The figure shows three views and two pictorial views of one solid part (mm, origin at its lowest corner). Answer the questions. Give positions to 0.01 mm unless a question says otherwise; leave off trailing zeros. Loops run counter-clockwise (first coordinate to the right, second up) from the corner with the lowest first, then second, coordinate; pieces in that order, holes last. Notation, with made-up numbers: (69, 48.5) - (93, 48.5) arc R15 ccw to (93, 57.5) - close; hole circle Ø6 at (-24.75, -21). An arc over 180 degrees is marked (long way). Use a Markdown table: item, result. Add a question column.
Item 1: Consider probe 1 along Y at (x, z) = (10, 2.05); probe 2 along X at (y, z) = (6, 1.15); probe 3 along X at (y, z) = (5.5, 0.45). Determine where each line is inside the solid, lowest interval first. Write a range as [from, to].
Item 2: A cutting plane is placed at B-B (y = 1.5). Determine the outline of the cut face in (x, z), plus the area to 3 significant figures.
Item 3: This flat-tipped pin is pushed along its axis until it touches: P1, Ø1, axis at y = 8, z = 4, coming from the -X side. Where does it stop, or does it pass through?
Item 4: A cutting plane is placed at C-C (x = 10). Determine the outline of the cut face in (y, z), plus the area to 3 significant figures.
Item 5: A cutting plane is placed at A-A (z = 2.5). Determine the outline of the cut face in (x, y), plus the area to 3 significant figures.
Item 6: A cutting plane is placed at D-D (y = 4.85). Determine the outline of the cut face in (x, z), plus the area to 3 significant figures.
Item 7: For a pull along Y with two mould halves and no side action, classify the marked faces 1, 2, 3 and 4 as +Y half, -Y half, draft (parallel to the pull), parting line (faces both ways), or undercut.
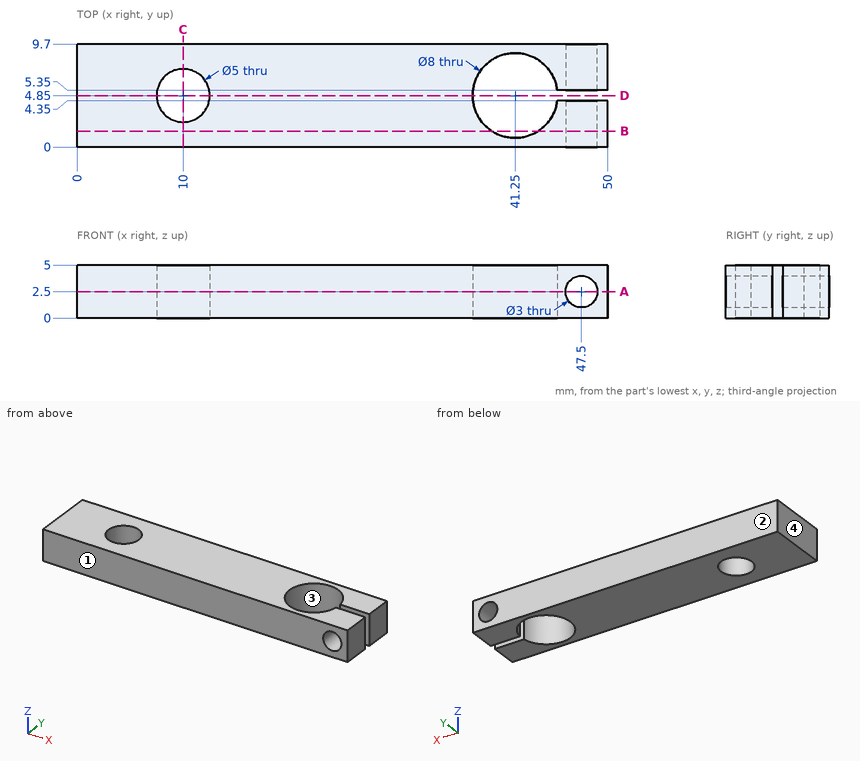
Geometry says:
| question | item | result |
|---|---|---|
| 1 | probe 1 | [0, 2.35], [7.35, 9.7] |
| 1 | probe 2 | [0, 7.78], [12.22, 37.42], [45.08, 46.85], [48.15, 50] |
| 1 | probe 3 | [0, 7.59], [12.41, 37.3], [45.2, 50] |
| 2 | outline | (0, 0) - (39.06, 0) - (39.06, 5) - (0, 5) - close; (43.44, 0) - (50, 0) - (50, 5) - (43.44, 5) - close; hole circle Ø3 at (47.5, 2.5) |
| 2 | area | 221 mm² |
| 3 | P1 | x = 0 |
| 4 | outline | (0, 0) - (2.35, 0) - (2.35, 5) - (0, 5) - close; (7.35, 0) - (9.7, 0) - (9.7, 5) - (7.35, 5) - close |
| 4 | area | 23.5 mm² |
| 5 | outline | (0, 0) - (46, 0) - (46, 4.35) - (45.22, 4.35) arc R4 cw (long way) to (45.22, 5.35) - (46, 5.35) - (46, 9.7) - (0, 9.7) - close; (49, 0) - (50, 0) - (50, 4.35) - (49, 4.35) - close; (49, 5.35) - (50, 5.35) - (50, 9.7) - (49, 9.7) - close; hole circle Ø5 at (10, 4.85) |
| 5 | area | 384 mm² |
| 6 | outline | (0, 0) - (7.5, 0) - (7.5, 5) - (0, 5) - close; (12.5, 0) - (37.25, 0) - (37.25, 5) - (12.5, 5) - close |
| 6 | area | 161 mm² |
| 7 | face 1 | -Y half |
| 7 | face 2 | +Y half |
| 7 | face 3 | undercut |
| 7 | face 4 | draft |
